```python
from build123d import *

# Parameters (mm, degrees)
SKETCH_1_R             = 35
EXTRUDE_1_DEPTH        = 38
SKETCH_2_W             = 12
SKETCH_2_H             = 15
EXTRUDE_2_DEPTH        = 11
SKETCH_3_R             = 2.95
EXTRUDE_3_DEPTH        = 63
HOLE_WIZARD_M4_1_D     = 3.3
HOLE_WIZARD_M4_1_DEPTH = 5
HOLE_WIZARD_M4_1_TIP   = 0.991420021


with BuildPart() as part:
    # 草图1 → 凸台-拉伸1 (new body)
    with BuildSketch(Plane.XY):
        Circle(SKETCH_1_R)
    extrude(amount=EXTRUDE_1_DEPTH)

    # 草图2 → 凸台-拉伸2 (add)
    with BuildSketch(Plane(origin=(0, 41.2, 0), x_dir=(1, 0, 0), z_dir=(0, 1, 0))):
        with Locations((0, -7.5)):
            Rectangle(SKETCH_2_W, SKETCH_2_H)
    extrude(amount=-EXTRUDE_2_DEPTH)

    # 草图3 → 凸台-拉伸3 (add)
    with BuildSketch(Plane(origin=(6, 0, 0), x_dir=(0, 0, -1), z_dir=(1, 0, 0))):
        with Locations((-7.405885861, 37.760893476)):
            Circle(SKETCH_3_R)
    extrude(amount=-EXTRUDE_3_DEPTH)

    # M4 螺纹孔的螺纹孔钻头1
    with Locations(Plane(origin=(-9.918584156, 27.251086003, 38), x_dir=(1, 0, 0), z_dir=(0, 0, 1))):
        with Locations((0, 0), (19.837168312, 0), (38.478008993, -32.286883155), (28.559424837, -49.466374853), (-8.722256525, -49.466374853), (-18.640840681, -32.286883155)):
            Hole(HOLE_WIZARD_M4_1_D / 2, depth=HOLE_WIZARD_M4_1_DEPTH)
            with Locations((0, 0, -(HOLE_WIZARD_M4_1_DEPTH + HOLE_WIZARD_M4_1_TIP / 2))):  # 118° drill point
                Cone(0, HOLE_WIZARD_M4_1_D / 2, HOLE_WIZARD_M4_1_TIP, mode=Mode.SUBTRACT)


solid = part.part
```
Part model, mm, in its own coordinate system. A direction names the side the tool comes from. Round coordinates to 2 decimals unless told otherwise and drop trailing zeros. Loops run counter-clockwise (first coordinate to the right, second up) from the corner with the lowest first, then second, coordinate; pieces in that order, holes last. Notation, with made-up numbers: (7, 61.5) -> (57, 61.5) arc R18 cw to (57, 80.5) -> close; hole circle Ø1 at (49, 20). An arc over 180 degrees is marked (long way). Use one line per item in the form item = value. Start each with the question number.
Item 1: Band-saw the part on A-A (z = 35.5). List the corners of the cut face in (x, y).
Item 2: Band-saw the part on B-B (x = 0). List the corners of the cut face in (y, z).
Item 3: Tool access for faces 1 (the flat face through (6, 38, 8)), 2 (the cylindrical face through (-19.528, -20.824, 35.465)), 3 (the flat face through (0, 4, 0)), 4 (the flat face through (0, 0, 38)), 5 (the cylindrical face through (-31.143, 35.144, 6.045)): list every direction of +Z, -Z, +X, -X, +Y, -Y with a clear straight run to the whole face (end or side of a thin tool).
Item 4: Drop flat-ended pins along their axis: pin 1 Ø2 at (x, z) = (17, 8) entering from +Y; pin 2 Ø7.5 at (y, z) = (36, 5.5) entering from +X; pin 3 Ø12 at (x, z) = (2.5, 30) entering from -Y. Give the stop position or say it passes through.
Item 5: Band-saw the part on D-D (y = 11). List the corners of the cut face in (x, z), plus the area to 3 significant figures.
Item 6: Drill centre lines: line 1 along Z through (x, y) = (-42.5, 37.5); line 2 along X through (y, z) = (-20.5, 31); line 3 along X through (y, z) = (23.5, 14). Where is each one in solid material? Low to high.
Item 7: Band-saw the part on C-C (z = 31). List the corners of the cut face in (x, y).
Item 8: Two-plate mould, pull along X, no slides. Class faces 6 (the conical face through (18.906, -22.325, 32.181)), 7 (the conical face through (10.19, 27.34, 32.18)), 8 (the flat face through (0, 41.2, 7)), 9 (the flat face through (-57, 38, 7)): released by +X, released by -X, zero draft, split by the parting line, or undercut.
Data:
q1.outline = circle Ø70 at (0, 0); hole circle Ø3.3 at (-28.56, -5.04); hole circle Ø3.3 at (-18.64, -22.22); hole circle Ø3.3 at (-9.92, 27.25); hole circle Ø3.3 at (9.92, 27.25); hole circle Ø3.3 at (18.64, -22.22); hole circle Ø3.3 at (28.56, -5.04)
q2.outline = (-35, 0) -> (41.2, 0) -> (41.2, 15) -> (35, 15) -> (35, 38) -> (-35, 38) -> close
q3.face_1 = +Z, -Z, +X, +Y
q3.face_2 = +Z
q3.face_3 = -Z, +X, -X, +Y, -Y
q3.face_4 = +Z, +X, -X, +Y, -Y
q3.face_5 = -X
q4.pin_1 = 31.13
q4.pin_2 = 13.6
q4.pin_3 = -35
q5.outline = (-33.23, 0) -> (33.23, 0) -> (33.23, 38) -> (-33.23, 38) -> close
q5.area = 2,530 mm^2
q6.line_1 = 4.47 to 10.34
q6.line_2 = -28.37 to 28.37
q6.line_3 = -25.94 to 25.94
q7.outline = circle Ø70 at (0, 0)
q8.face_6 = undercut
q8.face_7 = undercut
q8.face_8 = zero draft
q8.face_9 = released by -X
